Autodesk Inventor part; units mm, degrees
ref_plane "YZ Plane" through (0, 0, 0) normal (1, 0, 0) x (0, 1, 0)
ref_plane "XZ Plane" through (0, 0, 0) normal (0, 1, 0) x (-1, 0, 0)
ref_plane "XY Plane" through (0, 0, 0) normal (0, 0, 1) x (1, 0, 0)
sketch "Sketch2" plane through (0, 0, 0) normal (0, 1, 0) x (-1, 0, 0)
  line L0 (25, -35) -> (-25, -35)
  line L1 (-25, -35) -> (-25, 35)
  line L2 (25, 30) -> (25, -35)
  line L3 (25, -35) -> (-25, 35) construction
  line L4 (-25, -35) -> (25, 35) construction
  line L5 (12, 35) -> (-3, 35)
  line L6 (6.5, 35) -> (12, 35)
  line L7 (-3, 35) -> (-25, 35)
  line L8 (25, 35) -> (6.5, 35)
  line L9 (6.5, 35) -> (6.5, 30)
  line L10 (6.5, 30) -> (25, 30)
  line L11 (25, 30) -> (25, 35)
  line L12 (-22.5, 35) -> (-7.5, 35)
  line L13 (-7.5, 35) -> (-7.5, 41)
  line L14 (-7.5, 41) -> (-22.5, 41)
  line L15 (-22.5, 41) -> (-22.5, 35)
  point P0 (0, 0)
  point P1 (0, 0)
  point P2 (-7.5, 35)
  dimension "d0" = 50
  dimension "d1" = 70
  dimension "d16" = 18.5
  dimension "d17" = 5
  dimension "d58" = 2.5
  dimension "d59" = 15
  dimension "d60" = 6
extrude "Extrusion3" add sketch "Sketch2" along normal blind 6 contours L0 L1 L7 L5 L9 L10 L2 | L15 L14 L13 L7
fillet "Fillet1" radius 2 3 edges at (25, 3, -35) (-25, 3, -35) (25, 3, 35)
sketch "Sketch4" plane through (0, 6, 0) normal (0, 1, 0) x (1, 0, 0)
  circle A0 centre (-1.75, -8) radius 2.5
  line L0 (25, -33) -> (25, 33)
  circle A1 centre (-21.5, -12) radius 1.5
  line L1 (-25, 33) -> (-25, -30)
  circle A2 centre (18, -12) radius 2.5
  line L2 (-6.5, -35) -> (7.5, -35)
  point P0 (0, 0)
  dimension "d31" = 5
  dimension "d34" = 3
  dimension "d41" = 5
  dimension "d44" = 19.75
  dimension "d45" = 19.75
  dimension "d46" = 7
  dimension "d61" = 23
  dimension "d62" = 27
  dimension "d63" = 23
extrude "Extrusion10" cut sketch "Sketch4" against normal through all
properties part number "Pared_caja_reduccion_MDF"
Geometry: final body of the model. Coordinates: model frame, mm. A direction names the side the tool comes from. Coordinates: 2 decimals unless noted, no trailing zeros. Order: outer loops, then holes, each group sorted by start corner. A loop starts at its lowest first (then second) coordinate and runs counter-clockwise, first axis right, second up.
(1) Access query for faces 5 (the face through (-24.4, 3.04, -34.43)), 6 (the face through (-16, 3, 30)). Directions: +Z, -Z, +X, -X, +Y, -Y. A direction counts if a zero-diameter tool reaches every point of the face in a straight line with its end or side. Return the directions, or none.
(2) Section query C-C (z = 8). Return the cut outline in (x, y).
(3) Material intervals for probe 1 along X at (y, z) = (2.9, 12); probe 2 along Z at (x, y) = (-21.5, 2.8); probe 3 along Z at (x, y) = (-1.75, 1.95), sorted ascending.
(4) First-contact query: pin 1 (3 mm diameter, centred on x = 18, z = 12, fed in from -Y); pin 2 (3 mm diameter, centred on y = 2, z = 38, fed in from +X); pin 3 (5 mm diameter, centred on x = -21.5, z = 12, fed in from +Y); pin 4 (1.8 mm diameter, centred on y = 4, z = 39, fed in from -X). Flat tips, straight axial feed; report the tip coordinate or a pass-through.
(5) Section query A-A (x = 16.5). Return the cut outline in (y, z).
(6) Draft query along X for faces 1 (the face through (-23, 3, 12)), 2 (the face through (22.5, 3, 38)), 3 (the face through (0, 3, -35)), 4 (the face through (7.5, 3, 38)). Return one class per face: pulls with the +X half, pulls with the -X half, needs draft (parallel to the pull), parting line crosses it, or undercut.
(7) Section query D-D (x = -19). Return the cut outline in (y, z).
(8) Section query B-B (y = 4). Return the cut outline in (x, z), plus the area to 3 significant figures.
Solution:
1. face 5: -Z, -X, +Y, -Y
1. face 6: +Z, -X, +Y, -Y
2. outline: (-25, 0) - (-4.25, 0) - (-4.25, 6) - (-25, 6) - close; (0.75, 0) - (25, 0) - (25, 6) - (0.75, 6) - close
3. probe 1: x = -25 to -23, -20 to 15.5, 20.5 to 25
3. probe 2: z = -35 to 10.5, 13.5 to 30
3. probe 3: z = -35 to 5.5, 10.5 to 35
4. pin 1: passes through
4. pin 2: stops at x = 22.5
4. pin 3: stops at y = 6
4. pin 4: stops at x = 7.5
5. outline: (0, -35) - (6, -35) - (6, 10) - (0, 10) - close; (0, 14) - (6, 14) - (6, 41) - (0, 41) - close
6. face 1: undercut
6. face 2: pulls with the +X half
6. face 3: needs draft
6. face 4: pulls with the -X half
7. outline: (0, -35) - (6, -35) - (6, 30) - (0, 30) - close
8. outline: (-25, -33) arc R2 ccw to (-23, -35) - (23, -35) arc R2 ccw to (25, -33) - (25, 33) arc R2 ccw to (23, 35) - (22.5, 35) - (22.5, 41) - (7.5, 41) - (7.5, 35) - (-6.5, 35) - (-6.5, 30) - (-25, 30) - close; hole circle Ø3 at (-21.5, 12); hole circle Ø5 at (-1.75, 8); hole circle Ø5 at (18, 12)
8. area: 3,450 mm2
